Source: CAD feature listing. Evaluate the final solid. Frame: model axes, mm. Round coordinates to 2 decimals unless told otherwise and drop trailing zeros. Order: outer loops, then holes, each group sorted by start corner. A loop starts at its lowest first (then second) coordinate and runs counter-clockwise, first axis right, second up. Notation, with made-up numbers: (67, 44.5) -> (79, 44.5) arc R15 cw to (79, 58.5) -> close; hole circle Ø3 at (-38.5, 12). An arc over 180 degrees is marked (long way). One line per item, written item: value. Start each with the question number.
1) Ray query, L1, parallel to X at y = 38, z = -10; L2, parallel to X at y = 63, z = -4.5; L3, parallel to Y at x = 12.5, z = -16. Return the intervals inside material, ascending.
2) Pin query (flat end, axial travel): P1, Ø2, axis at y = 53.5, z = 5, coming from the +X side; P2, Ø12, axis at y = 42.5, z = -11.5, coming from the -X side; P3, Ø2, axis at x = 16.5, z = -11, coming from the -Y side. Return the tip coordinate at first contact, or that it passes through.
3) Mould query, pull axis X, two halves, no side actions, for faces 1 (the face through (6, 69.873, 0)), 2 (the face through (-10.19, 36.95, 12.83)). Classes: pulls with the +X half, pulls with the -X half, needs draft (parallel to the pull), parting line crosses it, or undercut.
4) Section A-A (y = 7.5). Return the cut outline in (x, z), and give its area (3 significant figures).
```python
from build123d import *

# Parameters (mm, degrees)
F3_DEPTH = 0.0254


with BuildPart() as f1:
    # F0 (on Top) → F1 (revolve)
    with BuildSketch(Plane.XY):
        with BuildLine():
            Line((6.5402514301, 69.8725463986), (6.5402514301, 1.6435814323))
            add(Edge.make_bspline(
                [(6.5402514301, 1.6435814323), (16.6055685907, 1.6237888089), (24.4864700581, 1.0951121643), (24.2117271912, 0)],
                knots=[0, 0, 0, 0, 0.7582969465, 0.7582969465, 0.7582969465, 0.7582969465], degree=3))
            add(Edge.make_bspline(
                [(25.5896002368, 0.5953258758), (24.9631976139, 0.4681905354), (24.4171222, 0.2947845137), (24.2117271912, 0)],
                knots=[0.3083695275, 0.3083695275, 0.3083695275, 0.3083695275, 0.5848021934, 0.5848021934, 0.5848021934, 0.5848021934], degree=3))
            ThreePointArc((25.5896002368, 0.5953258758), (27.050958138, 1.47703779), (27.624379952, 3.0845732447))
            Line((27.624379952, 3.0845732447), (27.624379952, 69.8725463986))
            ThreePointArc((27.624379952, 69.8725463986), (26.8804311762, 71.6685976229), (25.084379952, 72.4125463986))
            add(Edge.make_bspline(
                [(25.084379952, 72.4125463986), (24.711275029, 71.678932761), (24.5228062968, 70.0934224878), (23.9885225892, 69.8725463986)],
                knots=[0, 0, 0, 0, 0.3680062222, 0.3680062222, 0.3680062222, 0.3680062222], degree=3))
            add(Edge.make_bspline(
                [(23.9885225892, 69.8725463986), (23.8915327068, 69.8324501995), (23.783146815, 69.837324245), (23.6659098082, 69.8725463986)],
                knots=[0.3680062222, 0.3680062222, 0.3680062222, 0.3680062222, 0.4348113291, 0.4348113291, 0.4348113291, 0.4348113291], degree=3))
            Line((23.6659098082, 69.8725463986), (6.5402514301, 69.8725463986))
        make_face()
        with BuildLine():
            Line((23.9885225892, 69.8725463986), (23.6659098082, 69.8725463986))
            add(Edge.make_bspline(
                [(23.9885225892, 69.8725463986), (23.8915327068, 69.8324501995), (23.783146815, 69.837324245), (23.6659098082, 69.8725463986)],
                knots=[0.3680062222, 0.3680062222, 0.3680062222, 0.3680062222, 0.4348113291, 0.4348113291, 0.4348113291, 0.4348113291], degree=3))
        make_face()
    revolve(axis=Axis((6.5402514301, 35.7580639155, 0), (0, 1, 0)))

    # F2 (on face) → F3 (join)
    with BuildSketch(Plane(origin=(0, 69.8725463986, 0), x_dir=(-1, 0, 0), z_dir=(0, 1, 0))):
        with BuildLine():
            ThreePointArc((-3.4999095369, 12.8522840624), (-3.3524060249, 13.5768925878), (-3.4999095369, 14.3015011132))
            ThreePointArc((-3.4999095369, 14.3015011132), (-6.7963991448, 16.4044588849), (-10.0287375972, 14.2041718005))
            ThreePointArc((-10.0287375972, 14.2041718005), (-10.1516131859, 13.5282279315), (-10.0287375972, 12.8522840624))
            ThreePointArc((-10.0287375972, 12.8522840624), (-6.764323567, 12.3472555866), (-3.4999095369, 12.8522840624))
        make_face()
    extrude(amount=F3_DEPTH)


solid = f1.part
```
Findings:
1. L1: -12.02 to 25.1
1. L2: -14.06 to 27.14
1. L3: 0.53 to 69.87
2. P1: x = 27.24
2. P2: x = -13.81
2. P3: y = 0.84
3. face 1: undercut
3. face 2: parting line crosses it
4. outline: circle Ø42.17 at (6.54, 0)
4. area: 1,400 mm2
